Can you work these out from the model? Positions are in its coordinate system, mm. A direction names the side the tool comes from. Coordinates: 2 decimals unless noted, no trailing zeros. Loops run counter-clockwise (first coordinate to the right, second up) from the corner with the lowest first, then second, coordinate; pieces in that order, holes last.
```python
from build123d import *

# Parameters (mm, degrees)
CUT_EXTRUDE1_DEPTH = 1.3
CHAMFER1_SIZE      = 0.35
FILLET1_R          = 0.2


with BuildPart() as part:
    # Sketch1 → Revolve1 (revolve)
    with BuildSketch(Plane(origin=(0, 0, 0), x_dir=(0, 0, -1), z_dir=(1, 0, 0))):
        with BuildLine():
            Line((-0.38, 3.8), (0, 3.8))
            Line((0, 3.8), (0, 2))
            Line((0, 2), (10, 2))
            Line((10, 2), (10, 0))
            Line((10, 0), (-2.2, 0))
            Line((-2.2, 0), (-2.2, 1.9))
            ThreePointArc((-2.2, 1.9), (-1.437986341, 2.991755338), (-0.38, 3.8))
        make_face()
    revolve(axis=Axis((0, 0, -10), (0, 0, 1)))

    # Sketch2 → Cut-Extrude1 (cut)
    with BuildSketch(Plane.XY.offset(2.2)):
        Polygon((1.154700538, 0), (0.577350269, 1), (-0.577350269, 1), (-1.154700538, 0), (-0.577350269, -1), (0.577350269, -1), align=None)
    extrude(amount=-CUT_EXTRUDE1_DEPTH, mode=Mode.SUBTRACT)

    # Chamfer1
    chamfer1_edges = [part.edges().sort_by_distance(p)[0] for p in [
        (0, -2, -10),
    ]]
    chamfer(chamfer1_edges, length=CHAMFER1_SIZE)

    # Fillet1
    fillet1_edges = [part.edges().sort_by_distance(p)[0] for p in [
        (0, -2, 0),
    ]]
    fillet(fillet1_edges, radius=FILLET1_R)


solid = part.part
```
(1) I want a section at C-C on z = 0.75. Write out the boundary of the cut face in (x, y), then the cut area to 3 significant figures.
Check values:
outline: circle Ø7.15 at (0, 0)
area: 40.1 mm2
(2) I'm going to push flat-ended pins straight in: pin 1 (1 mm diameter, centred on x = 1, y = -2, fed in from +Z); pin 2 (0.9 mm diameter, centred on x = 0, z = 1.5, fed in from +Y); pin 3 (1.5 mm diameter, centred on x = -0.5, z = -1.5, fed in from +Y); pin 4 (2 mm diameter, centred on y = 1.5, z = -4.5, fed in from +X). Where does each tip first touch, or does it pass through?
Check values:
pin 1: stops at z = 2.2
pin 2: stops at y = 3.35
pin 3: stops at y = 2
pin 4: stops at x = 1.94
(3) I want a section at B-B on y = -2.75. Write out the boundary of the cut face in (x, z), then the cut area to 3 significant figures.
Check values:
outline: (-2.62, 0) - (2.62, 0) - (2.62, 0.38) arc R3.34 ccw to (-2.62, 0.38) - close
area: 6.65 mm2
(4) If I drill on probe 1 along Z at (x, y) = (0.25, 0.75); probe 2 along Y at (x, z) = (-0.25, -3.5); probe 3 along X at (y, z) = (-1.25, -9.5), over which ranges is the centre line in solid material (lowest first)?
Check values:
probe 1: z = -10 to 0.9
probe 2: y = -1.98 to 1.98
probe 3: x = -1.56 to 1.56
(5) If we mould it in two halves opening along Y, with no side actions, what happens to faces 4 (the cylindrical face through (-0.167, -3.796, 0.187)), 5 (the flat face through (0, 0, -10)), 6 (the flat face through (0, -1, 2))? For each: released by +Y, released by -Y, zero draft, split by the parting line, or undercut.
Check values:
face 4: split by the parting line
face 5: zero draft
face 6: undercut
(6) Which directions (+Z, -Z, +X, -X, +Y, -Y) give clear straight access to the entire face, cutting with the end or side of a thin tool? Please do faces 1 (the flat face through (0, 1, 2)), 2 (the flat face through (2, 2, 0)), 3 (the flat face through (1, -1, 2.2)).
Check values:
face 1: +Z
face 2: -Z
face 3: +Z, +X, -X, +Y, -Y
(7) I want a section at A-A on z = -5.75. Write out the boundary of the cut face in (x, y).
Check values:
outline: circle Ø4 at (0, 0)
